Model file for the job. Use its own axes, mm. A direction names the side the tool comes from. Coordinates: 2 decimals unless noted, no trailing zeros. Order: outer loops, then holes, each group sorted by start corner. A loop starts at its lowest first (then second) coordinate and runs counter-clockwise, first axis right, second up. Notation, with made-up numbers: (24, 85) -> (34, 85) arc R26 cw to (34, 119) -> close; hole circle Ø5 at (-37.5, 2.5). An arc over 180 degrees is marked (long way). Return JSON: item names as keys, results as strings. Group by question number.
1) Cut at B-B (x = 0). Write the cut outline in (y, z).
2) Pull direction Z, two halves, no side cores. Call faces 1 (the flat face through (-7, -35, -250)), 2 (the flat face through (467, -35, -3)), 3 (the flat face through (-467, -35, -3)), 4 (the flat face through (-110, -70, 4)): +Z half, -Z half, draft (parallel to the pull), parting line (faces both ways), or undercut.
3) Cut at A-A (z = -179). Write the cut outline in (x, y).
4) Which spindle directions (+Z, -Z, +X, -X, +Y, -Y) get a long thin tool onto all of the face, cutting with end or side? Do faces 5 (the cylindrical face through (-9.764, -267.2, 74.362)), 6 (the flat face through (-7, 0, 4)). Say none if no direction does.
5) Cut at C-C (y = -139). Write the cut outline in (x, z).
6) Cut at D-D (z = 0). Write the cut outline in (x, y).
7) Flat gauge pins, fed straight in: pin 1 (1 mm diameter, centred on x = 149, z = -174.5, fed in from -Y); pin 2 (0.5 mm diameter, centred on x = 467.5, z = -170.5, fed in from +Y); pin 3 (0.8 mm diameter, centred on x = 467.5, y = -32, fed in from -Z); pin 4 (1.1 mm diameter, centred on x = -467.5, y = -40, fed in from +Z). Where does each tip first touch, or does it go through?
8) Probe line 1 (Y direction, x = -343.5, z = 157.5); line 2 (X direction, y = -48, z = -12); line 3 (X direction, y = -197, z = -51.5). List the from-to ranges inside material, lowest first.
from build123d import *

# Parameters (mm, degrees)
F0_W     = 934
F0_H     = 500
F1_DEPTH = 70
F2_R     = 75
F3_DEPTH = 400
F4_W     = 62
F4_H     = 51.8
F5_DEPTH = 1


# Not quite as in the source:
# - a pattern or mirror of a feature is missing from the dataset's text; its kind, count and spacing are read off the source's solid


with BuildPart() as f1:
    # F0 (on Front) → F1 (new body)
    with BuildSketch(Plane.XZ):
        Rectangle(F0_W, F0_H)
    extrude(amount=F1_DEPTH)

    # F2 (on face) → F3 (join)
    with BuildSketch(Plane.XZ.offset(70)):
        Circle(F2_R)
    extrude(amount=F3_DEPTH)

    # F4 (on face) → F5 (join)
    with BuildSketch(Plane.YZ.offset(467)):
        with Locations((-35, 181.5)):
            Rectangle(F4_W, F4_H)
        with Locations((-35, -181.5)):
            Rectangle(F4_W, F4_H)
    f5 = extrude(amount=F5_DEPTH)

    # F5_copies: F5 across plane
    add(f5.mirror(Plane(origin=(0, 0, 0), x_dir=(0, 0, -1), z_dir=(-1, 0, 0))))


solid = f1.part
Answers below:
{
 "1": {"outline": "(-470, -75) -> (-70, -75) -> (-70, -250) -> (0, -250) -> (0, 250) -> (-70, 250) -> (-70, 75) -> (-470, 75) -> close"},
 "2": {"face 1": "-Z half", "face 2": "undercut", "face 3": "undercut", "face 4": "draft"},
 "3": {"outline": "(-468, -66) -> (-467, -66) -> (-467, -70) -> (467, -70) -> (467, -66) -> (468, -66) -> (468, -4) -> (467, -4) -> (467, 0) -> (-467, 0) -> (-467, -4) -> (-468, -4) -> close"},
 "4": {"face 5": "-Y", "face 6": "+Z, -Z, +X, -X, +Y"},
 "5": {"outline": "circle Ø150 at (0, 0)"},
 "6": {"outline": "(-467, -70) -> (-75, -70) -> (-75, -470) -> (75, -470) -> (75, -70) -> (467, -70) -> (467, 0) -> (-467, 0) -> close"},
 "7": {"pin 1": "stops at y = -70", "pin 2": "stops at y = -4", "pin 3": "stops at z = -207.4", "pin 4": "stops at z = 250"},
 "8": {"line 1": "y = -70 to 0", "line 2": "x = -467 to 467", "line 3": "x = -54.52 to 54.52"}
}
